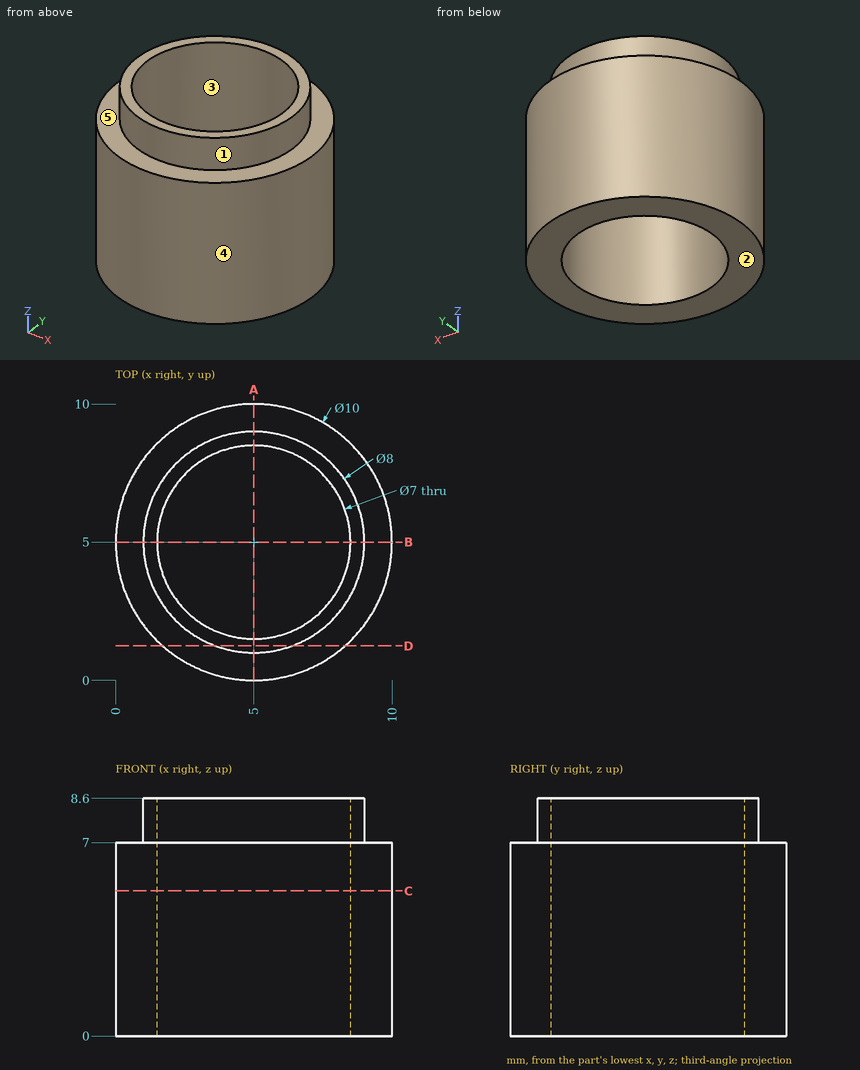
Print and shaded views of the part. All mm, measured from the part's lowest x, y and z. A direction names the side the tool comes from. Give positions to 0.01 mm unless a question says otherwise; leave off trailing zeros. Order: outer loops, then holes, each group sorted by start corner. A loop starts at its lowest first (then second) coordinate and runs counter-clockwise, first axis right, second up. Notation, with made-up numbers: M 34.5,56.5 L 73.5,56.5 A26 cw 73.5,86.5 Z; hole C 25,-13.5 d8. An arc over 180 degrees is marked long. Use one line per item in the form item = value.
Q1. Which spindle directions (+Z, -Z, +X, -X, +Y, -Y) get a long thin tool onto all of the face, cutting with end or side? Do the marked faces 4 and 5. Say none if no direction does.
Conclusion:
face_4 = +Z, -Z
face_5 = +Z
Q2. Slice it at D-D, the plane y = 1.25. Write the cut outline in (x, z), and give its area (3 significant figures).
Conclusion:
outline = M 1.69,0 L 8.31,0 L 8.31,7 L 6.39,7 L 6.39,8.6 L 3.61,8.6 L 3.61,7 L 1.69,7 Z
area = 50.8 mm2
Q3. Slice it at A-A, the plane x = 5. Write the cut outline in (y, z), and give its area (3 significant figures).
Conclusion:
outline = M 0,0 L 1.5,0 L 1.5,8.6 L 1,8.6 L 1,7 L 0,7 Z; M 8.5,0 L 10,0 L 10,7 L 9,7 L 9,8.6 L 8.5,8.6 Z
area = 22.6 mm2
Q4. Pin check, flat tip, straight feed: P1, Ø2, axis at y = 8, z = 1.5, coming from the +X side. Stop position of the tip, or through.
Conclusion:
P1 = 9.58
Q5. Pull direction X, two halves, no side cores. Call the marked faces 1, 2 and 3: released by +X, released by -X, zero draft, split by the parting line, or undercut.
Conclusion:
face_1 = split by the parting line
face_2 = zero draft
face_3 = undercut
Q6. Wall check: probe 1 along Y at (x, z) = (5, 2.25); probe 2 along Z at (x, y) = (1, 3); probe 3 along X at (y, z) = (8, 7.75). Give the ranges that are in metal, low to high.
Conclusion:
probe_1 = 0 to 1.5, 8.5 to 10
probe_2 = 0 to 7
probe_3 = 2.35 to 3.2, 6.8 to 7.65
Q7. Slice it at C-C, the plane z = 5.25. Write the cut outline in (x, y), and give its area (3 significant figures).
Conclusion:
outline = C 5,5 d10; hole C 5,5 d7
area = 40.1 mm2
